Design review of the part built by this model. Coordinates are the model's own, in mm. Face numbers are marked on the shaded views. A direction names the side the tool comes from. Round coordinates to 2 decimals unless told otherwise and drop trailing zeros. Write each loop counter-clockwise with the first axis right and the second up, starting at its lowest first coordinate (ties: lowest second). Pieces come first, ordered by that corner, then holes. Notation, with made-up numbers: M -27.75,55.5 L -15.75,55.5 A18 ccw -15.75,61.5 Z; hole C 85.25,40.25 d10. An arc over 180 degrees is marked long. One line per question, with ' | ' between items. Start each with the question number.
Item 1: For L1, parallel to Z at x = 13.75, y = 4.75; L2, parallel to X at y = 3.25, z = 3.5; L3, parallel to Y at x = 11.5, z = 5.75, list the stretches that pass through material, from the lowest coordinate up.
Item 2: Add section D-D, the plane z = 3.75. State the section outline as (x, y) points, and give its area (3 significant figures).
Item 3: Add section A-A, the plane x = 14. State the section outline as (y, z) points.
Item 4: Insertion check: pin 1 Ø2.5 at (x, z) = (10.5, 4) entering from -Y; pin 2 Ø4 at (x, z) = (18.5, 6.5) entering from -Y; pin 3 Ø1.8 at (x, y) = (11, 3) entering from +Z; pin 4 Ø0.5 at (x, z) = (10.5, 7.5) entering from -Y. Each pin has a flat end and moves straight along its axis. Give the tip position at first contact, or say it passes through.
Item 5: Machinability: for the marked faces 1 and 2, which of the approach directions +Z, -Z, +X, -X, +Y, -Y give a long, thin tool a straight path to every point of the face, cutting with its end or side? Answer none if there is none.
Item 6: Draft analysis for pull direction Z (two halves, no side actions). For the marked faces 3, 4, 5 and 6, state which applies: released by +Z, released by -Z, zero draft, split by the parting line, or undercut.
Item 7: Add section B-B, the plane y = 5.5. State the section outline as (x, z) points.
Item 8: Add section C-C, the plane y = 3.75. State the section outline as (x, z) points, and give its area (3 significant figures).
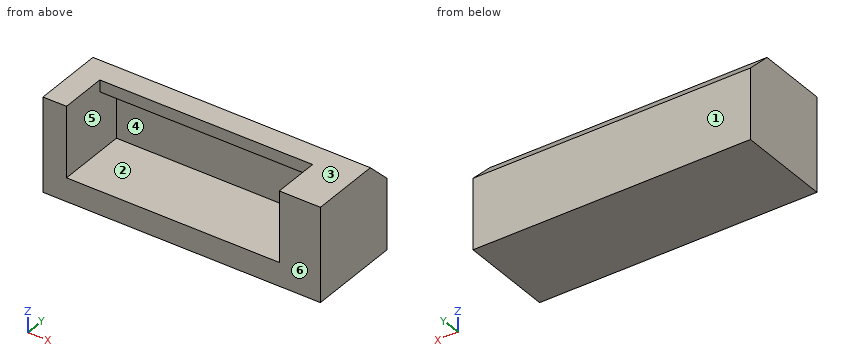
Autodesk Inventor part; units mm, degrees
ref_plane "РабПлоскость1" through (9.05, 0, 0) normal (1, 0, 0) x (0, 0, -1)
ref_plane "YZ Plane" through (0, 0, 0) normal (1, 0, 0) x (0, 1, 0)
ref_plane "XZ Plane" through (0, 0, 0) normal (0, 1, 0) x (-1, 0, 0)
sketch "Эскиз1" plane through (0, 0, 0) normal (0, 0, 1) x (1, 0, 0)
  line L0 (0, 0) -> (18.1, 0)
  line L1 (18.1, 0) -> (18.1, 8)
  line L2 (18.1, 8) -> (0, 8)
  line L3 (0, 8) -> (0, 0)
  dimension "d0" = 18.1
  dimension "d1" = 8
extrude "Выдавливание1" add sketch "Эскиз1" along normal blind 8
sketch "Эскиз2" plane through (0, 0, 8) normal (0, 0, 1) x (1, 0, 0)
  line L0 (0, 0) -> (18.1, 0)
  line L1 (18.1, 0) -> (18.1, 8)
  line L2 (0, 0) -> (18.1, 0)
  line L3 (18.1, 0) -> (18.1, 6)
  line L4 (18.1, 6) -> (0, 6)
  line L5 (0, 6) -> (0, 0)
  dimension "d4" = 6
extrude "Выдавливание2" cut sketch "Эскиз2" against normal blind 6
ref_plane "РабПлоскость1" through (9.05, 0, 0) normal (1, 0, 0) x (0, 0, -1)
sketch "Эскиз3" plane through (18.1, 0, 0) normal (1, 0, 0) x (0, 0, -1)
  line L0 (0, 8) -> (-8, 8)
  line L1 (0, 8) -> (0, 0)
  line L2 (-8, 8) -> (0, 8)
  line L3 (0, 8) -> (0, 0)
  line L4 (0, 0) -> (-8, 0)
  line L5 (-8, 0) -> (-8, 8)
extrude "Выдавливание3" add sketch "Эскиз3" along normal blind 3.5
chamfer "Фаска1" distance 2 angle 45 1 edges at (10.8, 8, 8)
sketch "Эскиз6" plane through (0, 6, 2) normal (0, -1, 0) x (1, 0, 0)
  line L0 (18.1, 6) -> (18.1, 0)
  line L1 (0, 6) -> (18.1, 6)
  line L2 (18.1, 6) -> (18.1, 5)
  line L3 (18.1, 5) -> (0, 5)
  line L4 (0, 5) -> (0, 6)
  line L5 (0, 0) -> (0, 6)
  point P0 (18, -2)
  dimension "d20" = 1
extrude "Выдавливание6" add sketch "Эскиз6" along normal blind 2
sketch "Эскиз7" plane through (0, 0, 0) normal (-1, 0, 0) x (0, 0, 1)
  line L0 (8, 6) -> (6, 8)
  line L1 (8, 6) -> (8, 0)
  line L2 (8, 0) -> (0, 0)
  line L3 (0, 0) -> (0, 8)
  line L4 (0, 8) -> (6, 8)
extrude "Выдавливание7" add sketch "Эскиз7" along normal blind 2
properties part number "Поворотный стоппер"
Computed values:
1) L1: z = 0 to 2, 7 to 8 | L2: x = -2 to 0, 18.1 to 21.6 | L3: y = 6 to 8
2) outline: M -2,0 L 0,0 L 0,6 L 18.1,6 L 18.1,0 L 21.6,0 L 21.6,8 L -2,8 Z | area: 80.2 mm^2
3) outline: M 0,0 L 8,0 L 8,6 L 6,8 L 4,8 L 4,7 L 6,7 L 6,2 L 0,2 Z
4) pin 1: stops at y = 6 | pin 2: stops at y = 0 | pin 3: stops at z = 2 | pin 4: stops at y = 4
5) face 1: +Z, -Z, +X, -X, +Y | face 2: -Y
6) face 3: released by +Z | face 4: undercut | face 5: undercut | face 6: zero draft
7) outline: M -2,0 L 21.6,0 L 21.6,8 L -2,8 Z; hole M 0,2 L 18.1,2 L 18.1,7 L 0,7 Z
8) outline: M -2,0 L 21.6,0 L 21.6,8 L 18.1,8 L 18.1,2 L 0,2 L 0,8 L -2,8 Z | area: 80.2 mm^2
